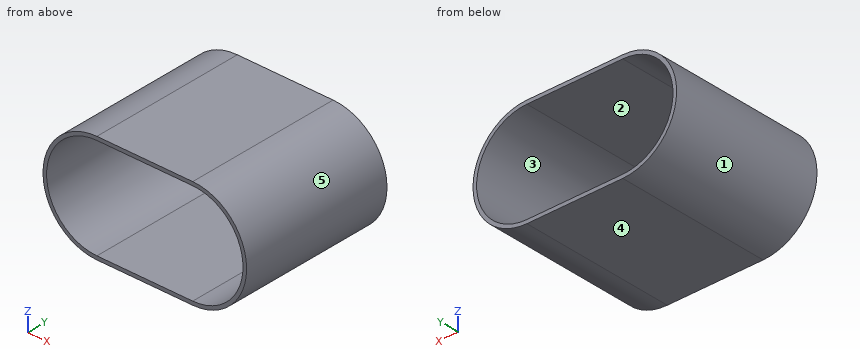
```python
from build123d import *

# Parameters (mm, degrees)
BOSS_EXTRUDE1_DEPTH = 130
SHELL1_T            = -3


with BuildPart() as part:
    # Sketch1 → Boss-Extrude1 (new body)
    with BuildSketch(Plane(origin=(0, 0, 0), x_dir=(1, 0, 0), z_dir=(0, 1, 0))):
        with BuildLine():
            Line((-40, -45), (40, -45))
            ThreePointArc((40, -45), (85, 0), (40, 45))
            Line((40, 45), (-40, 45))
            ThreePointArc((-40, 45), (-85, 0), (-40, -45))
        make_face()
    extrude(amount=BOSS_EXTRUDE1_DEPTH)

    # Shell1
    shell1_openings = [part.faces().sort_by_distance(p)[0] for p in [
        (0, 130, 0),
        (0, 0, 0),
    ]]
    offset(amount=SHELL1_T, openings=shell1_openings, kind=Kind.INTERSECTION)


solid = part.part
```
The listing builds one solid part. Answer for the finished solid, in the listing's coordinates (mm). Face numbers are marked on the shaded views. A direction names the side the tool comes from. Round coordinates to 2 decimals unless told otherwise and drop trailing zeros. Loops run counter-clockwise (first coordinate to the right, second up) from the corner with the lowest first, then second, coordinate; pieces in that order, holes last.
Q1. Given pin 1 Ø4 at (y, z) = (30.5, -14.5) entering from -X; pin 2 Ø1.5 at (y, z) = (63, 25.5) entering from +X, each flat-ended and moving along its own axis, determine where each tip first touches the part or whether it passes through.
Q2. Section C-C, the plane z = 0 is taken. Determine the outline of the cut face in (x, y).
Q3. For a pull along Z with two mould halves and no side action, classify the marked faces 3, 4 and 5 as released by +Z, released by -Z, zero draft, split by the parting line, or undercut.
Q4. Section B-B, the plane x = -10.5 is taken. Determine the outline of the cut face in (y, z).
Q5. Find the intervals of material crossed by line 1 (Z direction, x = -40, y = 91); line 2 (X direction, y = 119.5, z = -1); line 3 (X direction, y = 102, z = -27), in increasing order.
Q6. Which of the six approach directions +Z, -Z, +X, -X, +Y, -Y give full straight-line access (tool end or side, diameter ignored) to the marked faces 1 and 2?
Q7. Section A-A, the plane y = 97 is taken. Determine the outline of the cut face in (x, z), then the cut area to 3 significant figures.
Completed:
1. pin 1: stops at x = -83.23
1. pin 2: stops at x = 77.58
2. outline: (-85, 0) - (-82, 0) - (-82, 130) - (-85, 130) - close; (82, 0) - (85, 0) - (85, 130) - (82, 130) - close
3. face 3: undercut
3. face 4: released by -Z
3. face 5: split by the parting line
4. outline: (0, -45) - (130, -45) - (130, -42) - (0, -42) - close; (0, 42) - (130, 42) - (130, 45) - (0, 45) - close
5. line 1: z = -45 to -42, 42 to 45
5. line 2: x = -84.99 to -81.99, 81.99 to 84.99
5. line 3: x = -76 to -72.17, 72.17 to 76
6. face 1: -X, +Y, -Y
6. face 2: +Y, -Y
7. outline: (-40, -45) - (40, -45) arc R45 ccw to (40, 45) - (-40, 45) arc R45 ccw to start; hole (-40, -42) - (40, -42) arc R42 ccw to (40, 42) - (-40, 42) arc R42 ccw to start
7. area: 1,300 mm2
